from build123d import *

# Parameters (mm, degrees)
SKETCH1_R           = 12.5
BOSS_EXTRUDE1_DEPTH = 19
SKETCH2_R           = 12.1
BOSS_EXTRUDE2_DEPTH = 23
BOSS_EXTRUDE3_DEPTH = 2
SKETCH4_W           = 12
SKETCH4_H           = 4
BOSS_EXTRUDE4_DEPTH = 5
SKETCH5_R           = 3.5
BOSS_EXTRUDE5_DEPTH = 2.7
SKETCH6_R           = 2
BOSS_EXTRUDE6_DEPTH = 12.3
SKETCH7_R           = 1.5
CUT_EXTRUDE1_DEPTH  = 5


with BuildPart() as part:
    # Sketch1 → Boss-Extrude1 (new body)
    with BuildSketch(Plane.XY):
        Circle(SKETCH1_R)
    extrude(amount=BOSS_EXTRUDE1_DEPTH)

    # Sketch2 → Boss-Extrude2 (add)
    with BuildSketch(Plane.XY.offset(19)):
        Circle(SKETCH2_R)
    extrude(amount=BOSS_EXTRUDE2_DEPTH)

    # Sketch3 → Boss-Extrude3 (add)
    with BuildSketch(Plane.XY.offset(42)):
        with BuildLine():
            Line((-7, 17.9), (7, 17.9))
            Line((7, 17.9), (7, 9.86965045))
            ThreePointArc((7, 9.86965045), (0, -12.1), (-7, 9.86965045))
            Line((-7, 9.86965045), (-7, 17.9))
        make_face()
    extrude(amount=BOSS_EXTRUDE3_DEPTH)

    # Sketch4 → Boss-Extrude4 (add)
    with BuildSketch(Plane(origin=(0, 0, 42), x_dir=(-1, 0, 0), z_dir=(0, 0, -1))):
        with Locations((0, 14.9)):
            Rectangle(SKETCH4_W, SKETCH4_H)
    extrude(amount=BOSS_EXTRUDE4_DEPTH)

    # Sketch5 → Boss-Extrude5 (add)
    with BuildSketch(Plane(origin=(0, 0, 0), x_dir=(-1, 0, 0), z_dir=(0, 0, -1))):
        with Locations(Location((0, 0, 0), (0, 0, 180))):
            Circle(SKETCH5_R)
    extrude(amount=BOSS_EXTRUDE5_DEPTH)

    # Sketch6 → Boss-Extrude6 (add)
    with BuildSketch(Plane(origin=(0, 0, 0), x_dir=(-1, 0, 0), z_dir=(0, 0, -1))):
        Circle(SKETCH6_R)
    extrude(amount=BOSS_EXTRUDE6_DEPTH)

    # Sketch7 → Cut-Extrude1 (cut)
    with BuildSketch(Plane(origin=(0, 0, 0), x_dir=(-1, 0, 0), z_dir=(0, 0, -1))):
        with Locations((10, 0)):
            Circle(SKETCH7_R)
        with Locations((-10, 0)):
            Circle(SKETCH7_R)
    extrude(amount=-CUT_EXTRUDE1_DEPTH, mode=Mode.SUBTRACT)


solid = part.part
Here's how the part is built. I have some questions about the finished solid (model axes, mm). A direction names the side the tool comes from. Round coordinates to 2 decimals unless told otherwise and drop trailing zeros. Order: outer loops, then holes, each group sorted by start corner. A loop starts at its lowest first (then second) coordinate and runs counter-clockwise, first axis right, second up. Notation, with made-up numbers: M 15,-8 L 49,-8 A12 cw 49,7 Z; hole C 10,-31 d4. An arc over 180 degrees is marked long. One line per question, with ' | ' between items.
1) I need wall thicknesses on line 1 (Y direction, x = 0.5, z = 15.5); line 2 (Z direction, x = 4.5, y = 13); line 3 (Z direction, x = -0.5, y = -8). Which ranges of each line are inside material? Lowest first, please.
Checked values:
line 1: y = -12.49 to 12.49 | line 2: z = 37 to 44 | line 3: z = 0 to 44
2) We'd pull the mould along Y, two halves only. Please class faces 4 (the flat face through (-10, 0, 5)), 5 (the flat face through (2, 2, -2.7)), 6 (the cylindrical face through (0, -2, -7)): released by +Y, released by -Y, zero draft, split by the parting line, or undercut.
Checked values:
face 4: undercut | face 5: zero draft | face 6: split by the parting line
3) Imagine slicing it at A-A, the plane y = 0. Write out the boundary of the cut face in (x, z).
Checked values:
outline: M -12.5,0 L -11.5,0 L -11.5,5 L -8.5,5 L -8.5,0 L -3.5,0 L -3.5,-2.7 L -2,-2.7 L -2,-12.3 L 2,-12.3 L 2,-2.7 L 3.5,-2.7 L 3.5,0 L 8.5,0 L 8.5,5 L 11.5,5 L 11.5,0 L 12.5,0 L 12.5,19 L 12.1,19 L 12.1,44 L -12.1,44 L -12.1,19 L -12.5,19 Z
4) On a 3-axis mill with a long thin cutter (end or side, diameter ignored), from which of +Z, -Z, +X, -X, +Y, -Y can I reach the whole of each face in a straight line? I mean faces 1 (the flat face through (0, 16.9, 40)), 2 (the flat face through (-6, 15, 40)), 3 (the cylindrical face through (11.923, 3.755, 9.367)). Say none if no direction works.
Checked values:
face 1: -Z, +X, -X, +Y | face 2: -Z, -X, +Y | face 3: -Z
5) I'm going to push flat-ended pins straight in: pin 1 Ø0.9 at (x, y) = (9.5, 0.5) entering from -Z; pin 2 Ø1 at (x, z) = (5.5, 12) entering from +Y; pin 3 Ø6 at (x, z) = (5.5, 18) entering from +Y. Where does each tip first touch, or does it pass through?
Checked values:
pin 1: stops at z = 5 | pin 2: stops at y = 11.46 | pin 3: stops at y = 12.25
6) Imagine slicing it at B-B, the plane x = 0. Write out the boundary of the cut face in (y, z).
Checked values:
outline: M -12.5,0 L -3.5,0 L -3.5,-2.7 L -2,-2.7 L -2,-12.3 L 2,-12.3 L 2,-2.7 L 3.5,-2.7 L 3.5,0 L 12.5,0 L 12.5,19 L 12.1,19 L 12.1,42 L 12.9,42 L 12.9,37 L 16.9,37 L 16.9,42 L 17.9,42 L 17.9,44 L -12.1,44 L -12.1,19 L -12.5,19 Z
7) Imagine slicing it at C-C, the plane z = 17. Write out the boundary of the cut face in (x, y), plus the area to 3 significant figures.
Checked values:
outline: C 0,0 d25 | area: 491 mm²
8) Imagine slicing it at D-D, the plane y = -11. Write out the boundary of the cut face in (x, z), plus the area to 3 significant figures.
Checked values:
outline: M -5.94,0 L 5.94,0 L 5.94,19 L 5.04,19 L 5.04,44 L -5.04,44 L -5.04,19 L -5.94,19 Z | area: 478 mm²
